Job drawing, mm, ordinate dimensions from the low corner. One solid piece. Give positions to 0.01 mm unless a question says otherwise; leave off trailing zeros. Write each loop counter-clockwise with the first axis right and the second up, starting at its lowest first coordinate (ties: lowest second). Pieces come first, ordered by that corner, then holes. Notation, with made-up numbers: (52, 55.5) -> (89, 55.5) arc R25 cw to (89, 79.5) -> close; hole circle Ø4 at (-0.5, 55). An arc over 180 degrees is marked (long way). One line per question, with ' | ' between items. Start each with the question number.
(1) Band-saw the part on D-D, the plane x = 0.7. Give the cut face in (y, z), and give its area (3 significant figures).
(2) Band-saw the part on B-B, the plane z = 47.5. Give the cut face in (x, y), and give its area (3 significant figures).
(3) Band-saw the part on C-C, the plane y = 60. Give the cut face in (x, z), and give its area (3 significant figures).
(4) Band-saw the part on A-A, the plane y = 50. Give the cut face in (x, z), and give its area (3 significant figures).
(5) Pin check, flat tips, straight feed: P1, Ø4, axis at y = 17.5, z = 43, coming from the -X side; P2, Ø3, axis at y = 60, z = 12.5, coming from the -X side; P3, Ø1.5, axis at x = 1.5, z = 29.5, coming from the -Y side. Stop position of each tip, or through.
(6) Drill centre lines: probe 1 along Z at (x, y) = (1, 9.5); probe 2 along Y at (x, z) = (1.1, 12.5); probe 3 along Z at (x, y) = (0.8, 60.5). Where is each one in solid material? Low to high. Write a range as from..to.
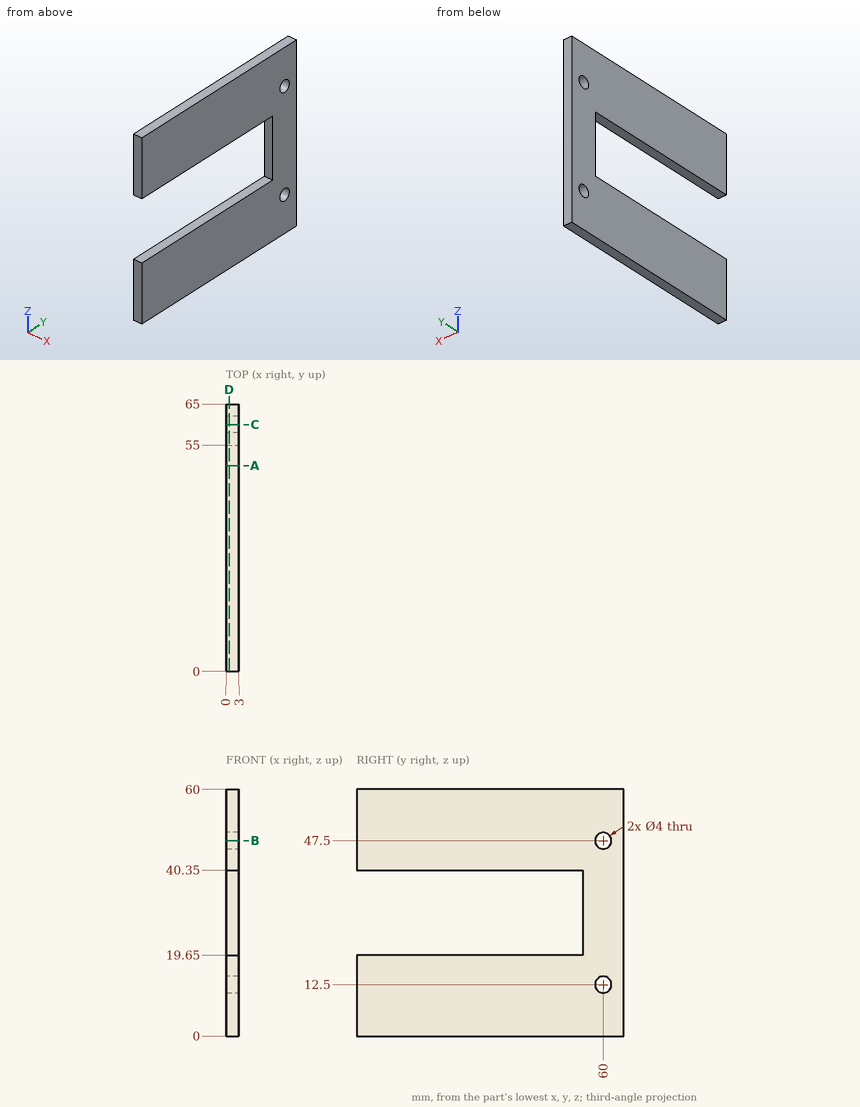
Results:
1) outline: (0, 0) -> (65, 0) -> (65, 60) -> (0, 60) -> (0, 40.35) -> (55, 40.35) -> (55, 19.65) -> (0, 19.65) -> close; hole circle Ø4 at (60, 12.5); hole circle Ø4 at (60, 47.5) | area: 2,740 mm²
2) outline: (0, 0) -> (3, 0) -> (3, 58) -> (0, 58) -> close; (0, 62) -> (3, 62) -> (3, 65) -> (0, 65) -> close | area: 183 mm²
3) outline: (0, 0) -> (3, 0) -> (3, 10.5) -> (0, 10.5) -> close; (0, 14.5) -> (3, 14.5) -> (3, 45.5) -> (0, 45.5) -> close; (0, 49.5) -> (3, 49.5) -> (3, 60) -> (0, 60) -> close | area: 156 mm²
4) outline: (0, 0) -> (3, 0) -> (3, 19.65) -> (0, 19.65) -> close; (0, 40.35) -> (3, 40.35) -> (3, 60) -> (0, 60) -> close | area: 118 mm²
5) P1: stops at x = 0 | P2: passes through | P3: stops at y = 55
6) probe 1: z = 0..19.65, 40.35..60 | probe 2: y = 0..58, 62..65 | probe 3: z = 0..10.56, 14.44..45.56, 49.44..60
